Design review of the part built by this model. Coordinates are the model's own, in mm. Face numbers are marked on the shaded views. A direction names the side the tool comes from. Give positions to 0.01 mm unless a question says otherwise; leave off trailing zeros. Loops run counter-clockwise (first coordinate to the right, second up) from the corner with the lowest first, then second, coordinate; pieces in that order, holes last. Notation, with made-up numbers: (6.5, 80) -> (61.5, 80) arc R33 cw to (61.5, 117) -> close; hole circle Ø8 at (-24, 76). An arc over 180 degrees is marked (long way). Use CSV: the item, a comma, the result in double quotes. Start each with the question number.
Item 1: We need section D-D (z = 0). State the section outline as (x, y) points.
Item 2: We need section B-B (x = -6.5). State the section outline as (y, z) points.
Item 3: For the marked faces 5, 6, 7 and 8, list the 3-axis set-ups (+Z, -Z, +X, -X, +Y, -Y) from which the entire face can be reached by the end or side of a thin tool; tool diameter is ignored.
Item 4: The part is to be moulded in two halves that separate along Y. For the marked faces 1, 2, 3 and 4, say which applies: +Y half, -Y half, draft (parallel to the pull), parting line (faces both ways), or undercut.
Item 5: Clearance check with flat-ended pins moving along their axes: pin 1 (10 mm diameter, centred on y = -43, z = 30, fed in from +X); pin 2 (5 mm diameter, centred on x = 37.5, y = 2, fed in from +Z); pin 3 (12 mm diameter, centred on x = -16, z = -3, fed in from -Y). State where each tip first meets the part, or that it passes through.
Item 6: We need section C-C (y = -35). State the section outline as (x, z) points, plus the area to 4 significant figures.
Item 7: Wall thickness on line 1 along Y through (x, z) = (0, 28.75); line 2 along Z through (x, y) = (27.5, -33.5); line 3 along Y through (x, z) = (0, 24): over which ranges is each line inside the solid? List them lowest first. Write a range as from..to.
Item 8: We need section A-A (y = -18.5). State the section outline as (x, z) points.
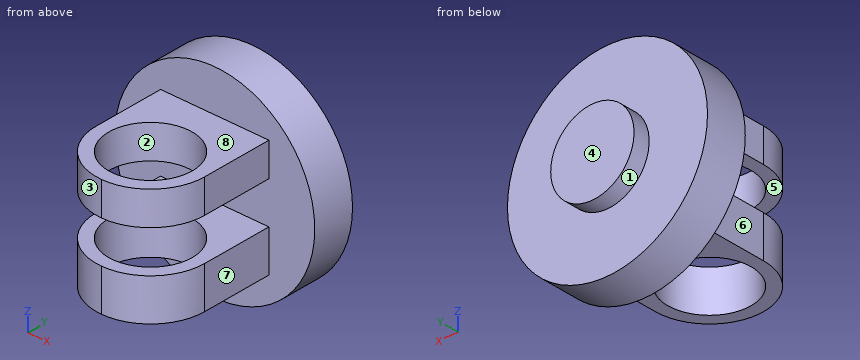
Autodesk Inventor part; units mm, degrees
ref_plane "YZ Plane" through (0, 0, 0) normal (1, 0, 0) x (0, 1, 0)
ref_plane "XZ Plane" through (0, 0, 0) normal (0, 1, 0) x (-1, 0, 0)
ref_plane "XY Plane" through (0, 0, 0) normal (0, 0, 1) x (1, 0, 0)
sketch "Sketch1" plane through (0, 0, 0) normal (0, 1, 0) x (-1, 0, 0)
  circle A0 centre (0, 0) radius 60
  dimension "d0" = 120
extrude "Extrusion1" add sketch "Sketch1" along normal mid plane 25
sketch "Sketch2" plane through (0, 12.5, 0) normal (0, 1, 0) x (1, 0, 0)
  circle A0 centre (0, 0) radius 60
  circle A1 centre (0, 0) radius 25
  dimension "d3" = 50
extrude "Extrusion2" add sketch "Sketch2" along normal blind 10 contours A1
sketch "Sketch3" plane through (0, -12.5, 0) normal (0, -1, 0) x (1, 0, 0)
  line L0 (32.5, 35) -> (-32.5, 35)
  line L1 (-32.5, 35) -> (-32.5, -35)
  line L2 (-32.5, -35) -> (32.5, -35)
  line L3 (32.5, -35) -> (32.5, 35)
  line L4 (32.5, 35) -> (-32.5, -35) construction
  line L5 (-32.5, 35) -> (32.5, -35) construction
  line L6 (32.5, 35) -> (-32.5, 35)
  line L7 (-32.5, 35) -> (-32.5, 15)
  line L8 (-32.5, 15) -> (32.5, 15)
  line L9 (32.5, 15) -> (32.5, 35)
  line L10 (32.5, -35) -> (-32.5, -35)
  line L11 (-32.5, -35) -> (-32.5, -10)
  line L12 (-32.5, -10) -> (32.5, -10)
  line L13 (32.5, -10) -> (32.5, -35)
  point P0 (0, 0)
  dimension "d6" = 65
  dimension "d7" = 70
  dimension "d8" = 20
  dimension "d9" = 25
extrude "Extrusion3" add sketch "Sketch3" along normal blind 75 contours L3 L8 L1 L0 | L3 L2 L1 L12
fillet "Fillet1" radius 32.5 4 edges at (32.5, -87.5, 25) (-32.5, -87.5, 25) (-32.5, -87.5, -22.5) (32.5, -87.5, -22.5)
sketch "Sketch4" plane through (-32.5, -12.5, 35) normal (0, 0, 1) x (1, 0, 0)
  circle A0 centre (32.5, -42.5) radius 25
  arc A1 (0, -42.5) -> (65, -42.5) centre (32.5, -42.5) ccw
  point P0 (32.5, 12.5)
  dimension "d13" = 50
extrude "Extrusion4" cut sketch "Sketch4" against normal blind 112.75
properties part number "JOINT BASE1"
Results found:
1,outline,"(-60, -12.5) -> (60, -12.5) -> (60, 12.5) -> (25, 12.5) -> (25, 22.5) -> (-25, 22.5) -> (-25, 12.5) -> (-60, 12.5) -> close"
2,outline,"(-86.84, -35) -> (-79.14, -35) -> (-79.14, -10) -> (-86.84, -10) -> close; (-86.84, 15) -> (-79.14, 15) -> (-79.14, 35) -> (-86.84, 35) -> close; (-30.86, -35) -> (-12.5, -35) -> (-12.5, -59.65) -> (12.5, -59.65) -> (12.5, -24.14) -> (22.5, -24.14) -> (22.5, 24.14) -> (12.5, 24.14) -> (12.5, 59.65) -> (-12.5, 59.65) -> (-12.5, 35) -> (-30.86, 35) -> (-30.86, 15) -> (-12.5, 15) -> (-12.5, -10) -> (-30.86, -10) -> close"
3,face 5,"+X, -X, -Y"
3,face 6,"+Z, -Z, -X, -Y"
3,face 7,"+Z, -Z, +X, -Y"
3,face 8,"+Z, +X, -X, -Y"
4,face 1,"draft"
4,face 2,"undercut"
4,face 3,"-Y half"
4,face 4,"+Y half"
5,pin 1,"x = 32.5"
5,pin 2,"z = 48.73"
5,pin 3,"y = -12.5"
6,outline,"(-32.5, -35) -> (-15, -35) -> (-15, -10) -> (-32.5, -10) -> close; (-32.5, 15) -> (-15, 15) -> (-15, 35) -> (-32.5, 35) -> close; (15, -35) -> (32.5, -35) -> (32.5, -10) -> (15, -10) -> close; (15, 15) -> (32.5, 15) -> (32.5, 35) -> (15, 35) -> close"
6,area,"1,575 mm²"
7,line 1,"-87.5..-80, -30..12.5"
7,line 2,"-35..-10, 15..35"
7,line 3,"-87.5..-80, -30..22.5"
8,outline,"(-32.5, -35) -> (32.5, -35) -> (32.5, -10) -> (-32.5, -10) -> close; (-32.5, 15) -> (32.5, 15) -> (32.5, 35) -> (-32.5, 35) -> close"
